Autodesk Inventor part; units mm, degrees
ref_plane "YZ Plane" through (0, 0, 0) normal (1, 0, 0) x (0, 1, 0)
ref_plane "XZ Plane" through (0, 0, 0) normal (0, 1, 0) x (-1, 0, 0)
ref_plane "XY Plane" through (0, 0, 0) normal (0, 0, 1) x (1, 0, 0)
sketch "Sketch1" plane through (0, 0, 0) normal (0, 0, 1) x (1, 0, 0)
  circle A0 centre (0, 0) radius 4.8
  arc A1 (-1.2481, -4.6349) -> (4.7694, 0.541) centre (0, 0) ccw
  circle A2 centre (0, 0) radius 9
  circle A3 centre (0, 0) radius 4.8
  circle A4 centre (0, 0) radius 7.5
  circle A5 centre (0, 0) radius 5.5
  point P0 (0, 0)
  dimension "d0" = 15
  dimension "d23" = 11
extrude "Extrusion1" add sketch "Sketch1" along normal blind 9 contours A4
sketch "Sketch2" plane through (0, 0, 9) normal (0, 0, 1) x (1, 0, 0)
  line L0 (4.7694, 0.541) -> (-1.2481, -4.6349)
  line L1 (-4.7694, -0.541) -> (1.2481, 4.6349)
  circle A0 centre (0, 0) radius 7.5
  line L2 (-5.478, -0.491) -> (1.3046, 5.343)
  line L3 (-2.0867, 2.426) -> (-5.478, -0.491)
  line L4 (-1.3046, -5.343) -> (5.478, 0.491)
  line L5 (2.0867, -2.426) -> (-0.6256, -4.7591)
  arc A1 (-5.478, -0.491) -> (-1.3046, -5.343) centre (0, 0) ccw
  arc A2 (5.478, 0.491) -> (1.3046, 5.343) centre (0, 0) ccw
extrude "Extrusion2" add sketch "Sketch2" along normal blind 34.2598
sketch "Sketch3" plane through (0, 0, 43.2598) normal (0, 0, 1) x (1, 0, 0)
  circle A0 centre (0, 0) radius 7.5
  circle A1 centre (0, 0) radius 7.5
  point P0 (0, 0)
extrude "Extrusion3" add sketch "Sketch3" along normal blind 2
sketch "Sketch5" plane through (0, 0, 45.2598) normal (0, 0, 1) x (1, 0, 0)
  circle A0 centre (0, 0) radius 4
  dimension "d10" = 8
extrude "Extrusion5" add sketch "Sketch5" along normal blind 5
sketch "Sketch6" plane through (0, 0, 50.2598) normal (0, 0, 1) x (1, 0, 0)
  circle A0 centre (0, 0) radius 4
  line L0 (-4, 0) -> (0, 4)
  line L1 (0, 4) -> (4, 0)
  line L2 (4, 0) -> (0, -4)
  line L3 (0, -4) -> (-4, 0)
extrude "Extrusion6" add sketch "Sketch6" along normal blind 16 contours L2 L3 L0 L1
sketch "Sketch7" plane through (0, 0, 66.2598) normal (0, 0, 1) x (1, 0, 0)
  circle A0 centre (0, 0) radius 2.8284
  line L0 (0, 4) -> (-4, 0)
extrude "Extrusion7" add sketch "Sketch7" along normal blind 8
sketch "Sketch8" plane through (0, 0, 9) normal (0, 0, -1) x (-1, 0, 0)
  point P0 (0, 0)
sketch "Sketch9" plane through (0, 0, 43.2598) normal (0, 0, -1) x (-1, 0, 0)
  line L0 (1.0362, -6.2993) -> (-6.5532, 0.2287)
  line L1 (6.1416, 0.1254) -> (-2.464, 7.5275)
  arc A0 (0.1057, -5.499) -> (5.453, 0.7177) centre (0, 0) ccw
  arc A1 (-0.1057, 5.499) -> (-5.453, -0.7177) centre (0, 0) ccw
  point P0 (0, 0)
  point P1 (0, 0)
extrude "Extrusion8" cut sketch "Sketch9" along normal blind 50
sketch "Sketch10" plane through (0, 0, 43.2598) normal (0, 0, -1) x (-1, 0, 0)
  circle A0 centre (0, 0) radius 5.5
  dimension "d28" = 11
extrude "Extrusion9" cut sketch "Sketch10" along normal blind 50
sketch "Sketch11" plane through (0, 0, 43.2598) normal (0, 0, -1) x (-1, 0, 0)
  line L0 (-4.1828, 4.1) -> (4.1828, 4.1)
  line L1 (4.1828, -4.1) -> (-4.1828, -4.1)
  line L2 (-12.4976, 4.1) -> (12.4976, -4.1) construction
  line L3 (12.4976, 4.1) -> (-12.4976, -4.1) construction
  arc A0 (4.1828, 4.1) -> (-4.1828, 4.1) centre (0, 0) ccw
  arc A1 (-4.1828, -4.1) -> (4.1828, -4.1) centre (0, 0) ccw
  point P0 (0, 0)
  dimension "d34" = 8.2
extrude "Extrusion10" add sketch "Sketch11" along normal blind 39.4125
scale "Scale1" factors (0.5, 0.5, 0.5) then translate (0, 0, 11.3149) bodies 1
properties part number "MainGearShaft"
Design review of the part built by this model. Coordinates are the model's own, in mm. A direction names the side the tool comes from. Coordinates: 2 decimals unless noted, no trailing zeros. Loops run counter-clockwise (first coordinate to the right, second up) from the corner with the lowest first, then second, coordinate; pieces in that order, holes last. Notation, with made-up numbers: (-34.5, 6.5) - (11.5, 6.5) arc R19 ccw to (11.5, 27.5) - close; hole circle Ø2 at (-19, -35.75). An arc over 180 degrees is marked (long way). Use CSV: the item, a comma, the result in double quotes. Start each with the question number.
1) Consider section D-D on z = 40. Write out the cut boundary in (x, y), then the cut area to 3 significant figures.
2) For pin 1 Ø2 at (x, y) = (1.5, -2) entering from +Z; pin 2 Ø1.5 at (x, z) = (-1.5, 21.5) entering from +Y; pin 3 Ø1.5 at (y, z) = (2, 41.5) entering from -X, all flat-tipped, find the tip position at first contact; note any pin that passes through.
3) Consider section A-A on z = 46.5. Write out the cut boundary in (x, y), then the cut area to 3 significant figures.
4) Consider section C-C on z = 35. Write out the cut boundary in (x, y), then the cut area to 3 significant figures.
5) Wall thickness on L1, parallel to Y at x = 0, z = 18; L2, parallel to Z at x = 2.75, y = 2.25; L3, parallel to Z at x = -2, y = -1: over which ranges is each line inside the solid? List them lowest first. Write a range as from..to.
6) Tool access review of faces 1 (the flat face through (-1, 1, 40)), 2 (the flat face through (1, 1, 40)), 3 (the cylindrical face through (-0.31, 1.38, 46.42)), 4 (the cylindrical face through (-2.6, -0.9, 22.3)), 5 (the flat face through (1.14, -1.14, 36.445)): name each direction out of +Z, -Z, +X, -X, +Y, -Y from which nothing blocks a thin tool from reaching the whole face with its end or side.
7) The part is to be moulded in two halves that separate along Y. For faces 6 (the flat face through (0, 0, 32.945)), 7 (the flat face through (-1.2, -1.1, 36.445)), 8 (the flat face through (-1, -1, 40)), 9 (the flat face through (0, 2.05, 23)), say which applies: +Y half, -Y half, draft (parallel to the pull), parting line (faces both ways), or undercut.
Geometry says:
1,outline,"(-2, 0) - (0, -2) - (2, 0) - (0, 2) - close"
1,area,"8.00 mm^2"
2,pin 1,"z = 36.44"
2,pin 2,"y = 3.67"
2,pin 3,"x = -0.75"
3,outline,"circle Ø2.83 at (0, 0)"
3,area,"6.28 mm^2"
4,outline,"circle Ø4 at (0, 0)"
4,area,"12.6 mm^2"
5,L1,"-3.75..-2.05, 2.05..3.75"
5,L2,"11.31..33.94"
5,L3,"32.94..33.94"
6,face 1,"+Z, -X, +Y"
6,face 2,"+Z, +X, +Y"
6,face 3,"+Z"
6,face 4,"-Z"
6,face 5,"+Z, +X, -Y"
7,face 6,"undercut"
7,face 7,"draft"
7,face 8,"-Y half"
7,face 9,"undercut"
